Design review of the part built by this model. Coordinates are the model's own, in mm. A direction names the side the tool comes from. Coordinates: 2 decimals unless noted, no trailing zeros. Loops run counter-clockwise (first coordinate to the right, second up) from the corner with the lowest first, then second, coordinate; pieces in that order, holes last.
from build123d import *

# Parameters (mm, degrees)
F0_W      = 146.954681846
F0_H      = 50.8
F0_W_2    = 56.245318154
F1_DEPTH  = 12.7
F2_W      = 73.3197343707
F2_H      = 50.8
F3_DEPTH  = 25.4
F4_W      = 58.0222320914
F4_H      = 37.0360761881
F5_DEPTH  = 25.4
F7_DEPTH  = 6.35
F8_R      = 6.35
F9_W      = 22.0035612583
F9_H      = 5.7547800243
F10_DEPTH = 57.15
F11_R     = 6.35
F13_D     = 6.35


with BuildPart() as f1:
    # F0 (on Top) → F1 (new body)
    with BuildSketch(Plane.XY):
        with Locations((-28.122659077, 0)):
            Rectangle(F0_W, F0_H)
        with Locations((73.477340923, 0)):
            Rectangle(F0_W_2, F0_H)
    extrude(amount=F1_DEPTH)

    # F2 (on face) → F3 (join)
    with BuildSketch(Plane.XY.offset(12.7)):
        with Locations((64.9401328146, 0)):
            Rectangle(F2_W, F2_H)
    extrude(amount=F3_DEPTH)

    # F4 (on face) → F5 (cut)
    with BuildSketch(Plane.XY.offset(38.1)):
        with Locations((64.9401328146, 0)):
            Rectangle(F4_W, F4_H)
    extrude(amount=-F5_DEPTH, mode=Mode.SUBTRACT)

    # F6 (on face) → F7 (cut)
    with BuildSketch(Plane.XY.offset(12.7)):
        with BuildLine():
            Line((-37.7411283553, 19.2452520132), (-94.6118757129, 19.2452520132))
            ThreePointArc((-94.6118757129, 19.2452520132), (-98.5048138537, 15.3523138724), (-94.6118757129, 11.4593757316))
            Line((-94.6118757129, 11.4593757316), (-37.7411283553, 11.4593757316))
            ThreePointArc((-37.7411283553, 11.4593757316), (-33.8481902145, 15.3523138724), (-37.7411283553, 19.2452520132))
        make_face()
        with BuildLine():
            Line((-37.7411283553, 4.519790411), (-94.6118757129, 4.519790411))
            ThreePointArc((-94.6118757129, 4.519790411), (-98.8433300517, 0.2883360721), (-94.6118757129, -3.9431182668))
            Line((-94.6118757129, -3.9431182668), (-37.7411283553, -3.9431182668))
            ThreePointArc((-37.7411283553, -3.9431182668), (-33.5096740164, 0.2883360721), (-37.7411283553, 4.519790411))
        make_face()
        with BuildLine():
            Line((21.6684918851, -13.2523179054), (-94.6118757129, -13.2523179054))
            ThreePointArc((-94.6118757129, -13.2523179054), (-98.1662971899, -16.8067393824), (-94.6118757129, -20.3611608595))
            Line((-94.6118757129, -20.3611608595), (21.6684918851, -20.3611608595))
            ThreePointArc((21.6684918851, -20.3611608595), (25.2229133621, -16.8067393824), (21.6684918851, -13.2523179054))
        make_face()
    extrude(amount=-F7_DEPTH, mode=Mode.SUBTRACT)

    # F8
    f8_edges = [f1.edges().sort_by_distance(p)[0] for p in [
        (28.280266, -25.4, 25.4),
        (28.280266, 25.4, 25.4),
        (-101.6, -25.4, 6.35),
        (-101.6, 25.4, 6.35),
        (101.6, 25.4, 19.05),
        (101.6, -25.4, 19.05),
    ]]
    fillet(f8_edges, radius=F8_R)

    # F9 (on face) → F10 (join)
    with BuildSketch(Plane(origin=(28.2802656293, 0, 0), x_dir=(0, -1, 0), z_dir=(-1, 0, 0))):
        with Locations((-6.8131443113, 24.4069304317)):
            Rectangle(F9_W, F9_H)
    extrude(amount=F10_DEPTH)

    # F11
    f11_edges = [f1.edges().sort_by_distance(p)[0] for p in [
        (-28.869734, -4.188636, 24.40693),
        (-28.869734, 17.814925, 24.40693),
    ]]
    fillet(f11_edges, radius=F11_R)

    # F13 (through all)
    with Locations(Plane.XY.offset(27.2843204439)):
        with Locations((-16.899863258, 12.0606217533), (0, 12.0606217533), (18.3064360172, 12.0606217533), (18.3064360172, 0), (0, 0), (-16.899863258, 0)):
            Hole(F13_D / 2)


solid = f1.part
Q1. Machinability: for faces 4 (the flat face through (35.929, 0, 26)), 5 (the cylindrical face through (-19.93, 0.95, 6.26)), 6 (the cylindrical face through (-26.96, 16.004, 24.447)), which of the approach directions +Z, -Z, +X, -X, +Y, -Y give a long, thin tool a straight path to every point of the face, cutting with its end or side? Answer none if there is none.
Q2. Take a section at D-D, the plane z = 3. Write out the cut boundary in (x, y) (3 decimals).
Q3. Clearance check with flat-ended pins moving along their axes: pin 1 Ø1 at (y, z) = (8, 16.5) entering from -X; pin 2 Ø5 at (y, z) = (2, 27.5) entering from -X; pin 3 Ø7.5 at (x, y) = (-16.9, 0) entering from +Z. State where each tip first meets the part, or that it passes through.
Q4. Take a section at C-C, the plane x = -70.5. Write out the cut boundary in (y, z).
Q5. Take a section at B-B, the plane z = 30. Write out the cut boundary in (x, y).
Q6. Take a section at A-A, the plane x = -8. Write out the cut boundary in (y, z), then the cut area to 3 significant figures.
Q7. The part is to be moulded in two halves that separate along X. For faces 1 (the cylindrical face through (-33.51, 0.2, 9.57)), 2 (the flat face through (-101.6, 0, 6)), 3 (the flat face through (20, 25.4, 10)), say which applies: pulls with the +X half, pulls with the -X half, needs draft (parallel to the pull), parting line crosses it, or undercut.
Q8. For line 1 (Y direction, x = -70, z = 12); line 2 (Y direction, x = 0, z = 9.5) (3 decimals); line 3 (Y direction, x = 0, z = 25.05) (3 decimals), list the stretches that pass through material, from the lowest coordinate up.
Entries:
1. face 4: +Z
1. face 5: +Z, -Z
1. face 6: +Z, -X, +Y
2. outline: (-101.6, -19.05) arc R6.35 ccw to (-95.25, -25.4) - (95.25, -25.4) arc R6.35 ccw to (101.6, -19.05) - (101.6, 19.05) arc R6.35 ccw to (95.25, 25.4) - (-95.25, 25.4) arc R6.35 ccw to (-101.6, 19.05) - close; hole circle Ø6.35 at (-16.9, 0); hole circle Ø6.35 at (-16.9, 12.061); hole circle Ø6.35 at (0, 0); hole circle Ø6.35 at (0, 12.061); hole circle Ø6.35 at (18.306, 0); hole circle Ø6.35 at (18.306, 12.061)
3. pin 1: stops at x = 28.28
3. pin 2: stops at x = -28.87
3. pin 3: stops at z = 27.28
4. outline: (-25.4, 0) - (25.4, 0) - (25.4, 12.7) - (19.25, 12.7) - (19.25, 6.35) - (11.46, 6.35) - (11.46, 12.7) - (4.52, 12.7) - (4.52, 6.35) - (-3.94, 6.35) - (-3.94, 12.7) - (-13.25, 12.7) - (-13.25, 6.35) - (-20.36, 6.35) - (-20.36, 12.7) - (-25.4, 12.7) - close
5. outline: (28.28, -19.05) arc R6.35 ccw to (34.63, -25.4) - (95.25, -25.4) arc R6.35 ccw to (101.6, -19.05) - (101.6, 19.05) arc R6.35 ccw to (95.25, 25.4) - (34.63, 25.4) arc R6.35 ccw to (28.28, 19.05) - close; hole (35.93, -18.52) - (93.95, -18.52) - (93.95, 18.52) - (35.93, 18.52) - close
6. outline: (-25.4, 0) - (25.4, 0) - (25.4, 12.7) - (-13.25, 12.7) - (-13.25, 6.35) - (-20.36, 6.35) - (-20.36, 12.7) - (-25.4, 12.7) - close; (-4.19, 21.53) - (17.81, 21.53) - (17.81, 27.28) - (-4.19, 27.28) - close
6. area: 727 mm2
7. face 1: undercut
7. face 2: pulls with the -X half
7. face 3: needs draft
8. line 1: y = -25.4 to -20.36, -13.25 to -3.94, 4.52 to 11.46, 19.25 to 25.4
8. line 2: y = -25.4 to -20.361, -13.252 to -3.175, 3.175 to 8.886, 15.236 to 25.4
8. line 3: y = -4.189 to -3.175, 3.175 to 8.886, 15.236 to 17.815
